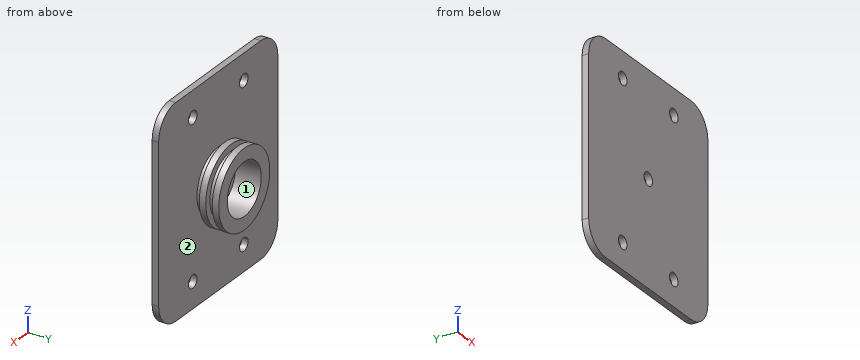
Autodesk Inventor part; units mm, degrees
ref_plane "YZ Plane" through (0, 0, 0) normal (1, 0, 0) x (0, 1, 0)
ref_plane "XZ Plane" through (0, 0, 0) normal (0, 1, 0) x (-1, 0, 0)
ref_plane "XY Plane" through (0, 0, 0) normal (0, 0, 1) x (1, 0, 0)
sketch "Sketch2" plane through (0, 0, 0) normal (0, 1, 0) x (-1, 0, 0)
  line L0 (-44.45, 50.8) -> (44.45, 50.8)
  line L1 (44.45, 50.8) -> (44.45, -50.8)
  line L2 (44.45, -50.8) -> (-44.45, -50.8)
  line L3 (-44.45, -50.8) -> (-44.45, 50.8)
  point P0 (0, 0)
  dimension "d0" = 44.45
  dimension "d1" = 44.45
  dimension "d2" = 50.8
  dimension "d3" = 50.8
extrude "Extrusion1" add sketch "Sketch2" along normal blind 3.175
fillet "Fillet1" radius 12.7 4 edges at (44.45, 1.5875, 50.8) (44.45, 1.5875, -50.8) (-44.45, 1.5875, 50.8) (-44.45, 1.5875, -50.8)
sketch "Sketch3" plane through (0, 3.175, 0) normal (0, 1, 0) x (1, 0, 0)
  line L0 (-44.45, -38.1) -> (-44.45, 38.1)
  line L1 (31.75, -50.8) -> (-31.75, -50.8)
  line L2 (44.45, 38.1) -> (44.45, -38.1)
  line L3 (-31.75, 50.8) -> (31.75, 50.8)
  point P0 (0, 0)
  point P1 (0, 0)
  point P2 (-19.05, 38.1)
  point P3 (19.05, 38.1)
  point P4 (19.05, -38.1)
  point P5 (-19.05, -38.1)
  dimension "d7" = 12.7
  dimension "d8" = 25.4
  dimension "d9" = 12.7
  dimension "d10" = 25.4
hole "Hole1" at (0, 3.175, 0) at (-19.05, 3.175, -38.1) at (19.05, 3.175, -38.1) at (19.05, 3.175, 38.1) at (-19.05, 3.175, 38.1) direction (0, -1, 0) diameter 6.35 end through all
sketch "Sketch4" plane through (0, 0, 0) normal (0, 0, 1) x (1, 0, 0)
  line L0 (12.7, 3.175) -> (12.7, 15.875)
  line L1 (12.7, 15.875) -> (19.05, 15.875)
  line L2 (19.05, 15.875) -> (19.05, 12.7)
  line L3 (19.05, 12.7) -> (15.875, 12.7)
  line L4 (15.875, 3.175) -> (12.7, 3.175)
  line L5 (15.875, 3.175) -> (12.7, 3.175)
  line L6 (15.875, 12.7) -> (15.875, 9.525)
  line L7 (15.875, 9.525) -> (19.05, 9.525)
  line L8 (19.05, 9.525) -> (19.05, 6.35)
  line L9 (19.05, 6.35) -> (15.875, 6.35)
  line L10 (15.875, 6.35) -> (15.875, 3.175)
  line L11 (15.875, 3.175) -> (12.7, 3.175)
  line L12 (0, -3.175) -> (0, 19.05)
  point P0 (0, 0)
  dimension "d18" = 12.7
  dimension "d19" = 6.35
  dimension "d20" = 3.175
  dimension "d21" = 3.175
  dimension "d22" = 9.525
  dimension "d23" = 12.7
  dimension "d24" = 3.175
  dimension "d25" = 3.175
  dimension "d26" = 3.175
  dimension "d27" = 3.175
  dimension "d28" = 3.175
revolve "Revolution1" add sketch "Sketch4" angle 360 about axis through (0, -10, 0) along (0, 1, 0)
equation "\"d4\" = metalThickness"
equation "\"metalThickness\" = 3.175"
properties part number "Rotation Base" material "Aluminum-6061"
The listing builds one solid part. Answer for the finished solid, in the listing's coordinates (mm). Face numbers are marked on the shaded views. Coordinates: 2 decimals unless noted, no trailing zeros. Write each loop counter-clockwise with the first axis right and the second up, starting at its lowest first coordinate (ties: lowest second). Pieces come first, ordered by that corner, then holes. Notation, with made-up numbers: (61, 73.25) - (73, 73.25) arc R35 ccw to (73, 110.25) - close; hole circle Ø2 at (-39, 78.25). An arc over 180 degrees is marked (long way). Return JSON: item names as keys, results as strings. Group by question number.
Q1. Flat-ended cylindrical pins translate along their axes: pin 1 Ø6 at (x, y) = (0.5, 9.5) entering from -Z; pin 2 Ø12.5 at (x, z) = (2.5, 4.5) entering from +Y (3 decimals); pin 3 Ø5 at (x, z) = (-19.05, 38.1) entering from +Y; pin 4 Ø1 at (x, y) = (-11, 4) entering from -Z. Find the tip coordinate at first contact, or state that the pin passes through.
Q2. The part is cut by section D-D on x = -29.5. Write down the section's boundary in (y, z) (3 decimals), and give its area (3 significant figures).
Q3. For a pull along X with two mould halves and no side action, classify the marked faces 1 and 2 as +X half, -X half, draft (parallel to the pull), parting line (faces both ways), or undercut.
Q4. The part is cut by section A-A on y = 7.5. Write down the section's boundary in (x, z).
Q5. The part is cut by section B-B on x = -8. Write down the section's boundary in (y, z) (3 decimals).
Q6. Find the intervals of material crossed by line 1 along Z through (x, y) = (-19.05, 1.65) (3 decimals); line 2 along X through (y, z) = (2.4, -38.1) (3 decimals); line 3 along Y through (x, z) = (-13, -10.5) (3 decimals), in increasing order. Write a range as [from, to].
Q7. The part is cut by section C-C on z = 44.5. Write down the section's boundary in (x, y) (1 decimal), and give its area (3 significant figures).
Evaluation:
{
 "1": {"pin 1": "stops at z = -19.05", "pin 2": "stops at y = 3.175", "pin 3": "passes through", "pin 4": "stops at z = -11.91"},
 "2": {"outline": "(0, -50.8) - (3.175, -50.8) - (3.175, 50.8) - (0, 50.8) - close", "area": "323 mm2"},
 "3": {"face 1": "undercut", "face 2": "draft"},
 "4": {"outline": "circle Ø38.1 at (0, 0); hole circle Ø25.4 at (0, 0)"},
 "5": {"outline": "(0, -50.8) - (3.175, -50.8) - (3.175, -13.712) - (6.35, -13.712) - (6.35, -17.289) - (9.525, -17.289) - (9.525, -13.712) - (12.7, -13.712) - (12.7, -17.289) - (15.875, -17.289) - (15.875, -9.864) - (3.175, -9.864) - (3.175, 9.864) - (15.875, 9.864) - (15.875, 17.289) - (12.7, 17.289) - (12.7, 13.712) - (9.525, 13.712) - (9.525, 17.289) - (6.35, 17.289) - (6.35, 13.712) - (3.175, 13.712) - (3.175, 50.8) - (0, 50.8) - close"},
 "6": {"line 1": "z = [-50.8, -41.275], [-34.925, 34.925], [41.275, 50.8]", "line 2": "x = [-44.45, -22.225], [-15.875, 15.875], [22.225, 44.45]", "line 3": "y = [0, 3.175], [6.35, 9.525], [12.7, 15.875]"},
 "7": {"outline": "(-42.7, 0) - (42.7, 0) - (42.7, 3.2) - (-42.7, 3.2) - close", "area": "271 mm2"}
}
